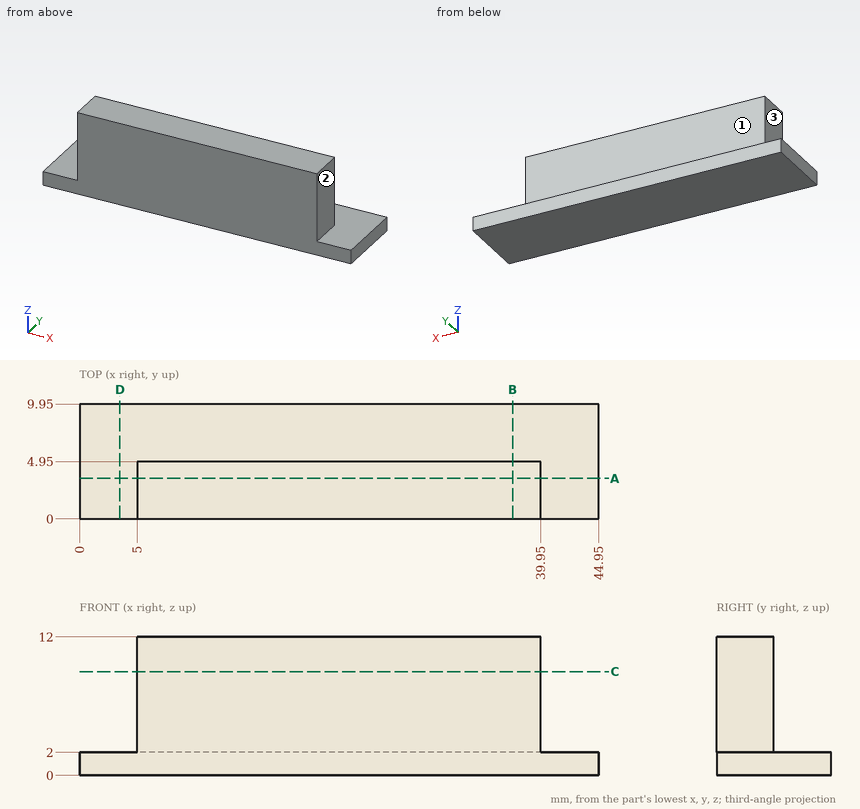
Verification items for this drawing (mm, ordinates from the low corner). A direction names the side the tool comes from. Coordinates: 2 decimals unless noted, no trailing zeros. Write each loop counter-clockwise with the first axis right and the second up, starting at its lowest first coordinate (ties: lowest second). Pieces come first, ordered by that corner, then holes. Notation, with made-up numbers: M 84.25,-14 L 107.25,-14 A9 ccw 107.25,-5 Z; hole C 70,88 d2. An arc over 180 degrees is marked long. Answer as a JSON object with one key per item and string values. Group by question number.
(1) Gauge pin test, flat ends, axial feed: pin 1 (3 mm diameter, centred on x = 22.5, z = 11, fed in from +Y); pin 2 (4 mm diameter, centred on y = 5, z = 5.5, fed in from -X); pin 3 (1 mm diameter, centred on y = 3.5, z = 9, fed in from +X). Record the tip position at first contact, or that the pin passes through.
(2) Tool access check on the marked faces 1, 2 and 3. Record the directions out of +Z, -Z, +X, -X, +Y, -Y that give a thin tool (end or side, any length) a straight path to the whole face; none if there is none.
(3) Cross-section at B-B, the plane x = 37.5. Record the cut outline in (y, z).
(4) Cross-section at A-A, the plane y = 3.5. Record the cut outline in (x, z), and give its area (3 significant figures).
(5) Cross-section at C-C, the plane z = 9. Record the cut outline in (x, y), and give its area (3 significant figures).
(6) Material ranges on line 1 (Z direction, x = 16.5, y = 5.25); line 2 (Y direction, x = 28, z = 5.25); line 3 (X direction, y = 3.5, z = 7.75), recorded low to high.
(7) Cross-section at D-D, the plane x = 3.5. Record the cut outline in (y, z).
Reply:
{
 "1": {"pin 1": "y = 4.95", "pin 2": "x = 5", "pin 3": "x = 39.95"},
 "2": {"face 1": "+Z, +X, -X, +Y", "face 2": "+Z, +X, +Y, -Y", "face 3": "+Z, -X, +Y, -Y"},
 "3": {"outline": "M 0,0 L 9.95,0 L 9.95,2 L 4.95,2 L 4.95,12 L 0,12 Z"},
 "4": {"outline": "M 0,0 L 44.95,0 L 44.95,2 L 39.95,2 L 39.95,12 L 5,12 L 5,2 L 0,2 Z", "area": "439 mm²"},
 "5": {"outline": "M 5,0 L 39.95,0 L 39.95,4.95 L 5,4.95 Z", "area": "173 mm²"},
 "6": {"line 1": "0 to 2", "line 2": "0 to 4.95", "line 3": "5 to 39.95"},
 "7": {"outline": "M 0,0 L 9.95,0 L 9.95,2 L 0,2 Z"}
}
